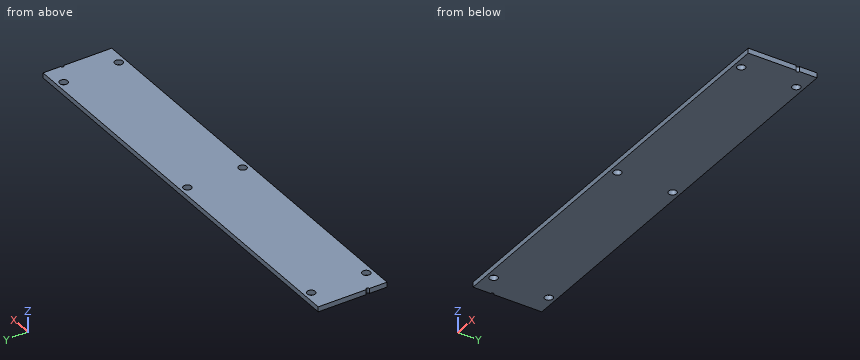
from build123d import *

# Parameters (mm, degrees)
SKETCH1_R           = 1.3125
BOSS_EXTRUDE1_DEPTH = 1.651


with BuildPart() as part:
    # Sketch1 → Boss-Extrude1 (new body)
    with BuildSketch(Plane.XY):
        with BuildLine():
            Line((-69.85, -5.5), (-69.85, -11.35))
            Line((-69.85, -11.35), (69.85, -11.35))
            Line((69.85, -11.35), (69.85, 4.5))
            ThreePointArc((69.85, 4.5), (69.35, 5), (69.85, 5.5))
            Line((69.85, 5.5), (69.85, 11.35))
            Line((69.85, 11.35), (-69.85, 11.35))
            Line((-69.85, 11.35), (-69.85, -4.5))
            ThreePointArc((-69.85, -4.5), (-69.496446609, -4.646446609), (-69.35, -5))
            ThreePointArc((-69.35, -5), (-69.496446609, -5.353553391), (-69.85, -5.5))
        make_face()
        with Locations(Location((-62.83, -9.1, 0), (0, 0, 180))):
            Circle(SKETCH1_R, mode=Mode.SUBTRACT)
        with Locations(Location((0, -9.1, 0), (0, 0, 180))):
            Circle(SKETCH1_R, mode=Mode.SUBTRACT)
        with Locations(Location((62.83, -9.1, 0), (0, 0, 180))):
            Circle(SKETCH1_R, mode=Mode.SUBTRACT)
        with Locations(Location((-62.83, 9.1, 0), (0, 0, 180))):
            Circle(SKETCH1_R, mode=Mode.SUBTRACT)
        with Locations(Location((0, 9.1, 0), (0, 0, 180))):
            Circle(SKETCH1_R, mode=Mode.SUBTRACT)
        with Locations(Location((62.83, 9.1, 0), (0, 0, 180))):
            Circle(SKETCH1_R, mode=Mode.SUBTRACT)
    extrude(amount=BOSS_EXTRUDE1_DEPTH)


solid = part.part
The model under review builds one solid part; all positions refer to its coordinate system, in mm. Give positions to 0.01 mm unless a question says otherwise; leave off trailing zeros. Order: outer loops, then holes, each group sorted by start corner. A loop starts at its lowest first (then second) coordinate and runs counter-clockwise, first axis right, second up. Notation, with made-up numbers: M 25.25,87 L 67.25,87 A28 cw 67.25,109 Z; hole C 24,-31.5 d7. An arc over 180 degrees is marked long. One line per question, with ' | ' between items. Start each with the question number.
1) Wall thickness on L1, parallel to X at y = -9.1, z = 0.55; L2, parallel to Y at x = -62.83, z = 0.9; L3, parallel to X at y = 9.75, z = 1.15: over which ranges is each line inside the solid? List them lowest first. Write a range as from..to.
2) Consider section B-B, the plane x = 0. Give the boundary of the cut face in (y, z), then the cut area to 3 significant figures.
3) Clearance check with a flat-ended pin moving along its axis: P1, Ø2, axis at x = 0, y = 9.1, coming from the -Z side. State where the tip first meets the part, or that it passes through.
4) Consider section A-A, the plane y = -9.1. Give the boundary of the cut face in (x, z), then the cut area to 3 significant figures.
Found:
1) L1: x = -69.85..-64.14, -61.52..-1.31, 1.31..61.52, 64.14..69.85 | L2: y = -11.35..-10.41, -7.79..7.79, 10.41..11.35 | L3: x = -69.85..-63.97, -61.69..-1.14, 1.14..61.69, 63.97..69.85
2) outline: M -11.35,0 L -10.41,0 L -10.41,1.65 L -11.35,1.65 Z; M -7.79,0 L 7.79,0 L 7.79,1.65 L -7.79,1.65 Z; M 10.41,0 L 11.35,0 L 11.35,1.65 L 10.41,1.65 Z | area: 28.8 mm²
3) P1: passes through
4) outline: M -69.85,0 L -64.14,0 L -64.14,1.65 L -69.85,1.65 Z; M -61.52,0 L -1.31,0 L -1.31,1.65 L -61.52,1.65 Z; M 1.31,0 L 61.52,0 L 61.52,1.65 L 1.31,1.65 Z; M 64.14,0 L 69.85,0 L 69.85,1.65 L 64.14,1.65 Z | area: 218 mm²
